from build123d import *

# Parameters (mm, degrees)
F1_DEPTH = 6.35
F2_R     = 12.7
F3_DEPTH = 10.16
F4_R     = 3.81
F5_DEPTH = 25.4


with BuildPart() as f1:
    # F0 (on Top) → F1 (new body)
    with BuildSketch(Plane.XY):
        Polygon((25.558257, -18.569161), (25.558257, 18.569161), (-9.762385, 30.045533), (-31.591743, 0), (-9.762385, -30.045533), align=None)
    extrude(amount=F1_DEPTH)

    # F2 (on face) → F3 (join)
    with BuildSketch(Plane.XY.offset(6.35)):
        Circle(F2_R)
        Polygon((0, 7.332348), (6.35, 3.666174), (6.35, -3.666174), (0, -7.332348), (-6.35, -3.666174), (-6.35, 3.666174), align=None, mode=Mode.SUBTRACT)
    extrude(amount=F3_DEPTH)

    # F4 (on face) → F5 (cut)
    with BuildSketch(Plane(origin=(0, 0, 0), x_dir=(1, 0, 0), z_dir=(0, 0, -1))):
        Circle(F4_R)
    extrude(amount=-F5_DEPTH, mode=Mode.SUBTRACT)


solid = f1.part
Can you work these out from the model? Positions are in its coordinate system, mm. A direction names the side the tool comes from. Coordinates: 2 decimals unless noted, no trailing zeros. Loops run counter-clockwise (first coordinate to the right, second up) from the corner with the lowest first, then second, coordinate; pieces in that order, holes last. Notation, with made-up numbers: (76, -13) - (90, -13) arc R25 ccw to (90, 26) - close; hole circle Ø2 at (3.25, 38.5). An arc over 180 degrees is marked (long way). Put each result on its own line as item: value. Start each with the question number.
Item 1: Suppose I cut it at D-D (y = -21). Please give me the cut outline in (x, z).
Item 2: If I drill on line 1 along X through (y, z) = (0, 2.75); line 2 along Z through (x, y) = (-23, 0.5); line 3 along Y through (x, z) = (-5, 10.5), over which ranges is the centre line in solid material (lowest first)?
Item 3: Suppose I cut it at C-C (z = 1.5). Please give me the cut outline in (x, y).
Item 4: Which directions (+Z, -Z, +X, -X, +Y, -Y) give clear straight access to the entire face, cutting with the end or side of a thin tool? Please do faces 4 (the face through (-3.131, -5.525, 11.359)), 5 (the face through (-0.83, 3.72, 3.13)).
Item 5: Suppose I cut it at A-A (z = 11.75). Please give me the cut outline in (x, y).
Item 6: For pin 1 (10 mm diameter, centred on x = -2.5, y = -2, fed in from +Z); pin 2 (5 mm diameter, centred on x = -24, z = 6, fed in from -Y); pin 3 (2 mm diameter, centred on x = -18, z = 3.5, fed in from -Y); pin 4 (1 mm diameter, centred on y = 21, z = 4, fed in from -X), each with a flat end and sliding along its axis, tell me the tip position at first contact or that it passes through.
Item 7: Suppose I cut it at B-B (x = 9.5). Please give me the cut outline in (y, z).
Item 8: If we mould it in two halves opening along X, with no side actions, what happens to faces 1 (the face through (-2.75, -12.4, 11.36)), 2 (the face through (25.558, 0, 3)), 3 (the face through (3, -3, 6.35))? For each: +X half, -X half, draft (parallel to the pull), parting line (faces both ways), or undercut.
Here are the results:
1. outline: (-16.33, 0) - (18.08, 0) - (18.08, 6.35) - (-16.33, 6.35) - close
2. line 1: -31.59 to -3.81, 3.81 to 25.56
2. line 2: 0 to 6.35
2. line 3: -11.67 to -4.45, 4.45 to 11.67
3. outline: (-31.59, 0) - (-9.76, -30.05) - (25.56, -18.57) - (25.56, 18.57) - (-9.76, 30.05) - close; hole circle Ø7.62 at (0, 0)
4. face 4: +Z
4. face 5: +Z, -Z
5. outline: circle Ø25.4 at (0, 0); hole (-6.35, -3.67) - (0, -7.33) - (6.35, -3.67) - (6.35, 3.67) - (0, 7.33) - (-6.35, 3.67) - close
6. pin 1: z = 16.51
6. pin 2: y = -13.89
6. pin 3: y = -20.08
6. pin 4: x = -16.7
7. outline: (-23.79, 0) - (23.79, 0) - (23.79, 6.35) - (8.43, 6.35) - (8.43, 16.51) - (-8.43, 16.51) - (-8.43, 6.35) - (-23.79, 6.35) - close
8. face 1: parting line
8. face 2: +X half
8. face 3: undercut
